Check sheet for the modelled part. Datum: model origin and axes. Units: mm. A direction names the side the tool comes from. Coordinates: 2 decimals unless noted, no trailing zeros. Write each loop counter-clockwise with the first axis right and the second up, starting at its lowest first coordinate (ties: lowest second). Pieces come first, ordered by that corner, then holes. Notation, with made-up numbers: (-13, 36) -> (-9, 36) arc R26 ccw to (-9, 55) -> close; hole circle Ø3 at (63.25, 47.5). An arc over 180 degrees is marked (long way). One line per item, written item: value. Start each with the question number.
1) Scan lines: line 1 along Y through (x, z) = (24.5, 0.9) (3 decimals); line 2 along X through (y, z) = (-28.5, 0.25); line 3 along X through (y, z) = (0, 0.2). Record each from-to range of solid material in increasing order. Write a range as [from, to].
2) Sectioned sample at C-C on z = 1. Give the number of separate pieces and of enclosed holes in the cut face, plus the area to 3 significant figures.
3) Set-up check for faces 1 (the flat face through (35, -15, 0)), 2 (the flat face through (33.6, -33, 0)), 3 (the flat face through (-35, -22.5, 0)), 4 (the flat face through (-33.6, -33, 0)), 5 (the flat face through (-33.6, 12, 0)): record each of +Z, -Z, +X, -X, +Y, -Y from which the full face is reachable in a straight line by a thin tool's end or side.
4) Sectioned sample at D-D on y = 2.5. Enter the section's corners in (x, z), plus the area to 3 significant figures.
5) Gauge pin test, flat ends, axial feed: P1, Ø0.9, axis at y = 13, z = 0.5, coming from the -X side; P2, Ø1.5, axis at y = -24, z = -0.5, coming from the +X side; P3, Ø1.5, axis at x = -36, z = -0.5, coming from the -Y side; P4, Ø3, axis at x = -24.5, y = 29, coming from the +Z side. Record the tip position at first contact, or that the pin passes through.
6) Sectioned sample at A-A on y = -29. Enter the section's corners in (x, z) (3 decimals), plus the area to 3 significant figures.
7) Sectioned sample at B-B on x = 24.5. Enter the section's corners in (y, z) (3 decimals).
8) Draft check along Y on faces 6 (the flat face through (-35, -27.5, 0)), 7 (the flat face through (-35, -10, 0)), 8 (the flat face through (-35, -15, 0)). Enter one of: +Y half, -Y half, draft (parallel to the pull), parting line (faces both ways), or undercut.
```python
from build123d import *

# Parameters (mm, degrees)
F0_R     = 1.375
F1_DEPTH = 1.5


with BuildPart() as f1:
    # F0 (on Top) → F1 (new body, symmetric)
    with BuildSketch(Plane.XY):
        with BuildLine():
            Line((33.6, 34.073957), (27.8, 34.073957))
            Line((27.8, 34.073957), (-27.8, 34.073957))
            Line((-27.8, 34.073957), (-33.6, 34.073957))
            Line((-33.6, 34.073957), (-33.6, -10))
            Line((-33.6, -10), (-36.8, -10))
            Line((-36.8, -10), (-36.8, -15))
            Line((-36.8, -15), (-33.6, -15))
            Line((-33.6, -15), (-33.6, -22.5))
            Line((-33.6, -22.5), (-36.8, -22.5))
            Line((-36.8, -22.5), (-36.8, -27.5))
            Line((-36.8, -27.5), (-33.6, -27.5))
            Line((-33.6, -27.5), (-33.6, -39.3))
            Line((-33.6, -39.3), (-27.8, -39.3))
            Line((-27.8, -39.3), (-27.8, -42.5))
            Line((-27.8, -42.5), (-12.8, -42.5))
            Line((-12.8, -42.5), (-12.8, -39.3))
            add(Edge.make_bspline(
                [(-12.8, -39.3), (-8.533333, -35.9), (0, -29.1), (8.533333, -35.9), (12.8, -39.3)],
                knots=[0, 0, 0, 0, 14.494137, 28.988273, 28.988273, 28.988273, 28.988273], degree=3))
            Line((12.8, -39.3), (12.8, -42.5))
            Line((12.8, -42.5), (27.8, -42.5))
            Line((27.8, -42.5), (27.8, -39.3))
            Line((27.8, -39.3), (33.6, -39.3))
            Line((33.6, -39.3), (33.6, -27.5))
            Line((33.6, -27.5), (36.8, -27.5))
            Line((36.8, -27.5), (36.8, -22.5))
            Line((36.8, -22.5), (33.6, -22.5))
            Line((33.6, -22.5), (33.6, -15))
            Line((33.6, -15), (36.8, -15))
            Line((36.8, -15), (36.8, -10))
            Line((36.8, -10), (33.6, -10))
            Line((33.6, -10), (33.6, -2.5))
            Line((33.6, -2.5), (36.8, -2.5))
            Line((36.8, -2.5), (40, -2.5))
            Line((40, -2.5), (40, 7.073957))
            Line((40, 7.073957), (36.8, 7.073957))
            Line((36.8, 7.073957), (36.8, 16.073957))
            Line((36.8, 16.073957), (40, 16.073957))
            Line((40, 16.073957), (40, 25.073957))
            Line((40, 25.073957), (36.8, 25.073957))
            Line((36.8, 25.073957), (36.8, 34.073957))
            Line((36.8, 34.073957), (33.6, 34.073957))
        make_face()
        with Locations((-24.5, -29)):
            Circle(F0_R, mode=Mode.SUBTRACT)
        with Locations((24.5, -29)):
            Circle(F0_R, mode=Mode.SUBTRACT)
        with Locations((-24.5, 29)):
            Circle(F0_R, mode=Mode.SUBTRACT)
        with Locations((24.5, 29)):
            Circle(F0_R, mode=Mode.SUBTRACT)
    extrude(amount=F1_DEPTH, both=True)


solid = f1.part
```
Answers:
1. line 1: y = [-42.5, -30.375], [-27.625, 27.625], [30.375, 34.074]
1. line 2: x = [-33.6, -25.78], [-23.22, 23.22], [25.78, 33.6]
1. line 3: x = [-33.6, 40]
2. separate pieces: 1
2. enclosed holes: 4
2. area: 5,130 mm2
3. face 1: +Z, -Z, +X
3. face 2: +Z, -Z, +X, -Y
3. face 3: +Z, -Z, -X
3. face 4: +Z, -Z, -X, -Y
3. face 5: +Z, -Z, -X, +Y
4. outline: (-33.6, -1.5) -> (40, -1.5) -> (40, 1.5) -> (-33.6, 1.5) -> close
4. area: 221 mm2
5. P1: stops at x = -33.6
5. P2: stops at x = 36.8
5. P3: stops at y = -27.5
5. P4: stops at z = 1.5
6. outline: (-33.6, -1.5) -> (-25.875, -1.5) -> (-25.875, 1.5) -> (-33.6, 1.5) -> close; (-23.125, -1.5) -> (23.125, -1.5) -> (23.125, 1.5) -> (-23.125, 1.5) -> close; (25.875, -1.5) -> (33.6, -1.5) -> (33.6, 1.5) -> (25.875, 1.5) -> close
6. area: 185 mm2
7. outline: (-42.5, -1.5) -> (-30.375, -1.5) -> (-30.375, 1.5) -> (-42.5, 1.5) -> close; (-27.625, -1.5) -> (27.625, -1.5) -> (27.625, 1.5) -> (-27.625, 1.5) -> close; (30.375, -1.5) -> (34.074, -1.5) -> (34.074, 1.5) -> (30.375, 1.5) -> close
8. face 6: -Y half
8. face 7: +Y half
8. face 8: undercut
